CAD build for the part. Positions are in the model's coordinates, mm. Give positions to 0.01 mm unless a question says otherwise; leave off trailing zeros. Write each loop counter-clockwise with the first axis right and the second up, starting at its lowest first coordinate (ties: lowest second). Pieces come first, ordered by that corner, then holes. Notation, with made-up numbers: M 62,-34.75 L 71,-34.75 A22 cw 71,4.25 Z; hole C -23.5,7.25 d8. An arc over 180 degrees is marked long. One line per question, with ' | ' between items. Start each with the question number.
1. Cut at A-A, the plane z = 242.5. Write the cut outline in (x, y), then the cut area to 3 significant figures.
2. Pull direction Y, two halves, no side cores. Call faces 1 (the face through (2.3, 27.1, 212)), 2 (the face through (-69.85, -61, 212)), 3 (the face through (-7.41, 34.61, 211.99)): released by +Y, released by -Y, zero draft, split by the parting line, or undercut.
3. Cut at B-B, the plane y = -18. Write the cut outline in (x, z).
4. Cut at C-C, the plane x = 11.5. Write the cut outline in (y, z).
5. Wall check: L1, parallel to Y at x = -12, z = 390.5; L2, parallel to X at y = -2.5, z = 406; L3, parallel to Y at x = -27, z = 327. Give the ranges that are in metal, low to high.
6. Flat gauge pins, fed straight in: pin 1 (2 mm diameter, centred on x = -29.5, z = 111.5, fed in from -Y); pin 2 (4 mm diameter, centred on y = 17, z = 189, fed in from -X); pin 3 (3 mm diameter, centred on x = 18.5, z = 61.5, fed in from +Y). Where does each tip first touch, or does it go through?
Autodesk Inventor part; units mm, degrees
ref_plane "YZ Plane" through (0, 0, 0) normal (1, 0, 0) x (0, 1, 0)
ref_plane "XZ Plane" through (0, 0, 0) normal (0, 1, 0) x (-1, 0, 0)
ref_plane "XY Plane" through (0, 0, 0) normal (0, 0, 1) x (1, 0, 0)
sketch "Sketch1" plane through (0, 0, 0) normal (0, 0, 1) x (1, 0, 0)
  line L0 (67.8086, 112.822) -> (-59.1914, -66.8193)
  line L1 (-69.85, 119.8) -> (69.85, 119.8)
  line L2 (67.8086, 119.8) -> (-65.0875, -68.2625)
  line L3 (-69.85, -61.8748) -> (-69.85, -68.2625)
  line L4 (-69.85, -68.2625) -> (-65.0875, -68.2625)
  line L5 (67.8086, 119.8) -> (53.3144, 119.8)
  line L6 (53.3144, 119.8) -> (-69.85, -52.9916)
  line L7 (-69.85, -52.9916) -> (-69.85, -61.8748)
  point P0 (0, 0)
extrude "Extrusion1" add sketch "Sketch1" along normal blind 430
properties part number "Backplane"
Here are the results:
1) outline: M -69.85,-68.26 L -65.09,-68.26 L 67.81,119.8 L 53.31,119.8 L -69.85,-52.99 Z | area: 2,750 mm^2
2) face 1: released by -Y | face 2: zero draft | face 3: released by +Y
3) outline: M -44.91,0 L -29.57,0 L -29.57,430 L -44.91,430 Z
4) outline: M 40.12,0 L 61.14,0 L 61.14,430 L 40.12,430 Z
5) L1: 6.86 to 28.17 | L2: -33.86 to -18.62 | L3: -14.36 to 7.12
6) pin 1: y = -19.32 | pin 2: x = -21.39 | pin 3: y = 73.06
